```python
from build123d import *

# Parameters (mm, degrees)
ESQUISSE3_R        = 32
ESQUISSE3_R_2      = 22.25
ESQUISSE3_R_3      = 1.925
BOSS_EXTRU_1_DEPTH = 5


with BuildPart() as part:
    # Esquisse3 → Boss.-Extru.1 (new body)
    with BuildSketch(Plane.XY):
        Circle(ESQUISSE3_R)
        Circle(ESQUISSE3_R_2, mode=Mode.SUBTRACT)
        with Locations((27.75, 0)):
            Circle(ESQUISSE3_R_3, mode=Mode.SUBTRACT)
        with Locations((-21.933137031, 17)):
            Circle(ESQUISSE3_R_3, mode=Mode.SUBTRACT)
        with Locations((-21.933137031, -17)):
            Circle(ESQUISSE3_R_3, mode=Mode.SUBTRACT)
    extrude(amount=BOSS_EXTRU_1_DEPTH)


solid = part.part
```
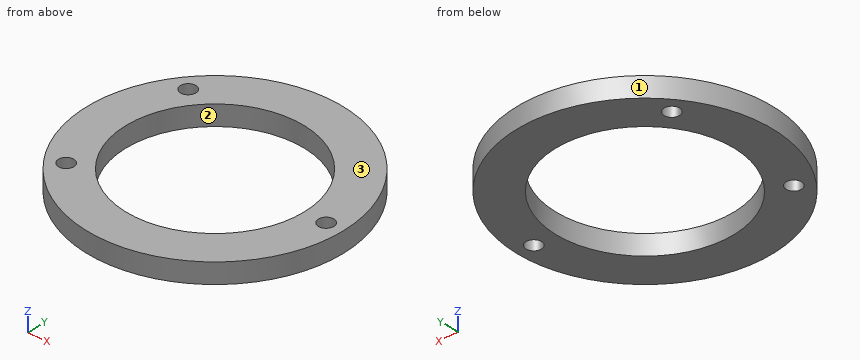
Source: CAD feature listing. Evaluate the final solid. Frame: model axes, mm. Face numbers are marked on the shaded views. Round coordinates to 2 decimals unless told otherwise and drop trailing zeros. Loops run counter-clockwise (first coordinate to the right, second up) from the corner with the lowest first, then second, coordinate; pieces in that order, holes last. Notation, with made-up numbers: M -1.75,2 L 41.25,2 A25 ccw 41.25,34 Z; hole C 5,73 d11. An arc over 180 degrees is marked long. Use a Markdown table: item, result. Add a question column.
1. Pull-direction query (X, two-part tool) for the marked faces 1, 2 and 3; classes: +X half, -X half, draft (parallel to the pull), parting line (faces both ways), or undercut.
2. Cut plane A-A, the plane x = 0. Output: boundary loops of the cut face in (y, z), and give its area (3 significant figures).
3. Cut plane D-D, the plane y = 17. Output: boundary loops of the cut face in (x, z), and give its area (3 significant figures).
4. Ray query, line 1 along Y through (x, z) = (0, 1.35); line 2 along X through (y, z) = (1, 2.45); line 3 along Y through (x, z) = (-23, 4.5). Return the intervals inside material, ascending. Write a range as [from, to].
5. Contact query for flat-ended pins moving along their axis: pin 1 (2 mm diameter, centred on y = -7, z = 3.5, fed in from -X); pin 2 (3 mm diameter, centred on x = 27.75, y = 0, fed in from -Z); pin 3 (1 mm diameter, centred on x = 20, z = 2.5, fed in from +Y). Output: stop coordinate, or through.
6. Cut plane B-B, the plane y = 0. Output: boundary loops of the cut face in (x, z) (3 decimals), and give its area (4 significant figures).
7. Cut plane C-C, the plane z = 1.55. Output: boundary loops of the cut face in (x, y) (3 decimals), and give its area (3 significant figures).
Solution:
| question | item | result |
|---|---|---|
| 1 | face 1 | parting line |
| 1 | face 2 | undercut |
| 1 | face 3 | draft |
| 2 | outline | M -32,0 L -22.25,0 L -22.25,5 L -32,5 Z; M 22.25,0 L 32,0 L 32,5 L 22.25,5 Z |
| 2 | area | 97.5 mm2 |
| 3 | outline | M -27.11,0 L -23.86,0 L -23.86,5 L -27.11,5 Z; M -20.01,0 L -14.35,0 L -14.35,5 L -20.01,5 Z; M 14.35,0 L 27.11,0 L 27.11,5 L 14.35,5 Z |
| 3 | area | 108 mm2 |
| 4 | line 1 | y = [-32, -22.25], [22.25, 32] |
| 4 | line 2 | x = [-31.98, -22.23], [22.23, 26.11], [29.39, 31.98] |
| 4 | line 3 | y = [-22.25, -18.6], [-15.4, 15.4], [18.6, 22.25] |
| 5 | pin 1 | stops at x = -31.43 |
| 5 | pin 2 | passes through |
| 5 | pin 3 | stops at y = 25.37 |
| 6 | outline | M -32,0 L -22.25,0 L -22.25,5 L -32,5 Z; M 22.25,0 L 25.825,0 L 25.825,5 L 22.25,5 Z; M 29.675,0 L 32,0 L 32,5 L 29.675,5 Z |
| 6 | area | 78.25 mm2 |
| 7 | outline | C 0,0 d64; hole C -21.933,-17 d3.85; hole C -21.933,17 d3.85; hole C 0,0 d44.5; hole C 27.75,0 d3.85 |
| 7 | area | 1,630 mm2 |
